from build123d import *

# Parameters (mm, degrees)
F1_DEPTH = 4
F2_DEPTH = 2


with BuildPart() as f1:
    # F0 (on Top) → F1 (new body)
    with BuildSketch(Plane.XY):
        with BuildLine():
            Line((0, 46), (0, 48.5))
            ThreePointArc((0, 48.5), (-43.2585399295, 21.9305431572), (-39.1209598697, -28.6670629621))
            Line((-39.1209598697, -28.6670629621), (-37.1044155465, -27.1893793042))
            ThreePointArc((-37.1044155465, -27.1893793042), (-41.0287182836, 20.8001027883), (0, 46))
        make_face()
        with BuildLine():
            ThreePointArc((-39.1209598697, -28.6670629621), (-0.384054582, -48.498479379), (38.6620589982, -29.2830188679))
            Line((38.6620589982, -29.2830188679), (36.6691693591, -27.7735849057))
            ThreePointArc((36.6691693591, -27.7735849057), (-0.3642579541, -45.9985577616), (-37.1044155465, -27.1893793042))
            Line((-37.1044155465, -27.1893793042), (-39.1209598697, -28.6670629621))
        make_face()
        with BuildLine():
            ThreePointArc((48.5, 0), (34.2946788875, 34.2946788875), (0, 48.5))
            Line((0, 48.5), (0, 46))
            ThreePointArc((0, 46), (32.5269119346, 32.5269119346), (46, 0))
            ThreePointArc((46, 0), (43.6049411794, -14.6495428168), (36.6691693591, -27.7735849057))
            Line((36.6691693591, -27.7735849057), (38.6620589982, -29.2830188679))
            ThreePointArc((38.6620589982, -29.2830188679), (45.9747749392, -15.445713622), (48.5, 0))
        make_face()
    extrude(amount=F1_DEPTH)

    # F0 (on Top) → F2 (join)
    with BuildSketch(Plane.XY):
        with BuildLine():
            Line((0, 48.5), (0, 50))
            ThreePointArc((-3e-10, 50), (-3.0000000001, 49.9099188539), (-5.9891902625, 49.64))
            ThreePointArc((-5.9891902625, 49.64), (-44.596432917, 22.6088073786), (-43.5805555109, -24.5098996604))
            ThreePointArc((-43.5805555109, -24.5098996604), (-42.0314458226, -27.0805753644), (-40.3308865052, -29.5536731))
            Line((-40.3308864636, -29.5536731568), (-39.1209598697, -28.6670629621))
            ThreePointArc((-39.1209598697, -28.6670629621), (-43.2585399295, 21.9305431572), (0, 48.5))
        make_face()
        with BuildLine():
            Line((0, 45), (0, 46))
            ThreePointArc((0, 46), (-41.0287182836, 20.8001027883), (-37.1044155465, -27.1893793042))
            Line((-37.1044155465, -27.1893793042), (-36.2977978173, -26.5983058411))
            ThreePointArc((-36.2977978173, -26.5983058411), (-40.1367896253, 20.3479266407), (0, 45))
        make_face()
        with BuildLine():
            ThreePointArc((35.9547017982, -34.7456388429), (37.9746633311, -32.5257581755), (39.8577928138, -30.1886792029))
            Line((39.8577927817, -30.1886792453), (38.6620589982, -29.2830188679))
            ThreePointArc((38.6620589982, -29.2830188679), (-0.384054582, -48.498479379), (-39.1209598697, -28.6670629621))
            Line((-39.1209598697, -28.6670629621), (-40.3308864636, -29.5536731568))
            ThreePointArc((-40.3308865052, -29.5536731), (-38.4850050472, -31.9202817425), (-36.5004526513, -34.1718737597))
            ThreePointArc((-36.5004526513, -34.1718737597), (-0.3959325588, -49.9984323495), (35.9547017982, -34.7456388429))
        make_face()
        with BuildLine():
            ThreePointArc((-37.1044155465, -27.1893793042), (-0.3642579541, -45.9985577616), (36.6691693591, -27.7735849057))
            Line((36.6691693591, -27.7735849057), (35.8720135035, -27.1698113208))
            ThreePointArc((35.8720135035, -27.1698113208), (-0.3563393029, -44.9985891146), (-36.2977978173, -26.5983058411))
            Line((-36.2977978173, -26.5983058411), (-37.1044155465, -27.1893793042))
        make_face()
        with BuildLine():
            ThreePointArc((-45.1705928336, -33.1001139433), (-41.0669741282, -35.5083498861), (-36.5004526513, -34.1718737597))
            ThreePointArc((-36.5004526513, -34.1718737597), (-38.4850050472, -31.9202817425), (-40.3308865052, -29.5536731))
            ThreePointArc((-40.3308865052, -29.5536731), (-39.8994627937, -30.3940375655), (-39.7507396514, -31.3268935462))
            ThreePointArc((-39.7507396514, -31.3268935462), (-41.8178836997, -34.1781704134), (-45.1705928336, -33.1001139433))
        make_face()
        with BuildLine():
            ThreePointArc((-39.7507396514, -31.3268935462), (-39.8994627937, -30.3940375655), (-40.3308865052, -29.5536731))
            ThreePointArc((-40.3308865052, -29.5536731), (-44.5239600731, -28.907040382), (-45.1705928336, -33.1001139433))
            ThreePointArc((-45.1705928336, -33.1001139433), (-41.8178836997, -34.1781704134), (-39.7507396514, -31.3268935462))
        make_face()
        with BuildLine():
            ThreePointArc((-40.7507396514, -31.3268935462), (-44.6515908972, -31.948797511), (-41.1375041929, -30.1447466199))
            ThreePointArc((-41.1375041929, -30.1447466199), (-40.8498884057, -30.7049895814), (-40.7507396514, -31.3268935462))
        make_face(mode=Mode.SUBTRACT)
        with BuildLine():
            ThreePointArc((-40.3308865052, -29.5536731), (-42.0314458226, -27.0805753644), (-43.5805555109, -24.5098996604))
            ThreePointArc((-43.5805555109, -24.5098996604), (-46.2306698509, -28.4616310409), (-45.1705928336, -33.1001139433))
            ThreePointArc((-45.1705928336, -33.1001139433), (-44.5239600731, -28.907040382), (-40.3308865052, -29.5536731))
        make_face()
        with BuildLine():
            ThreePointArc((44.640728683, -33.8113197413), (40.4379400794, -34.3914679346), (39.8577928138, -30.1886792029))
            ThreePointArc((39.8577928138, -30.1886792029), (37.9746633311, -32.5257581755), (35.9547017982, -34.7456388429))
            ThreePointArc((35.9547017982, -34.7456388429), (40.4994857112, -36.154266407), (44.640728683, -33.8113197413))
        make_face()
        with BuildLine():
            ThreePointArc((44.640728683, -33.8113197413), (45.774130629, -29.1902071747), (43.1869315491, -25.1970026665))
            ThreePointArc((43.1869315491, -25.1970026665), (41.597304838, -27.7428230397), (39.8577928138, -30.1886792029))
            ThreePointArc((39.8577928138, -30.1886792029), (43.2046653401, -29.1561994968), (45.2492603486, -32))
            ThreePointArc((45.2492603486, -32), (45.0930610627, -32.9554043637), (44.640728683, -33.8113197413))
        make_face()
        with BuildLine():
            ThreePointArc((45.2492603486, -32), (43.2046653401, -29.1561994968), (39.8577928138, -30.1886792029))
            ThreePointArc((39.8577928138, -30.1886792029), (40.4379400794, -34.3914679346), (44.640728683, -33.8113197413))
            ThreePointArc((44.640728683, -33.8113197413), (45.0930610627, -32.9554043637), (45.2492603486, -32))
        make_face()
        with BuildLine():
            ThreePointArc((44.2492603486, -32), (41.6123237043, -33.8958670078), (40.6549486373, -30.7924528302))
            ThreePointArc((40.6549486373, -30.7924528302), (42.8861969928, -30.1041329922), (44.2492603486, -32))
        make_face(mode=Mode.SUBTRACT)
        with BuildLine():
            ThreePointArc((43.1869315491, -25.1970026665), (48.2666892248, -13.050927602), (50, 0))
            ThreePointArc((50, 0), (37.4129624136, 33.1703217265), (5.9891902625, 49.64))
            ThreePointArc((5.9891902625, 49.64), (2.9999999999, 49.9099188539), (-3e-10, 50))
            Line((0, 50), (0, 48.5))
            ThreePointArc((0, 48.5), (34.2946788875, 34.2946788875), (48.5, 0))
            ThreePointArc((48.5, 0), (45.9747749392, -15.445713622), (38.6620589982, -29.2830188679))
            Line((38.6620589982, -29.2830188679), (39.8577927817, -30.1886792453))
            ThreePointArc((39.8577928138, -30.1886792029), (41.597304838, -27.7428230397), (43.1869315491, -25.1970026665))
        make_face()
        with BuildLine():
            ThreePointArc((46, 0), (32.5269119346, 32.5269119346), (0, 46))
            Line((0, 46), (0, 45))
            ThreePointArc((0, 45), (31.8198051534, 31.8198051534), (45, 0))
            ThreePointArc((45, 0), (42.6570076755, -14.3310744947), (35.8720135035, -27.1698113208))
            Line((35.8720135035, -27.1698113208), (36.6691693591, -27.7735849057))
            ThreePointArc((36.6691693591, -27.7735849057), (43.6049411794, -14.6495428168), (46, 0))
        make_face()
        with BuildLine():
            ThreePointArc((0, 56), (-3, 53.0000000001), (-3e-10, 50))
            ThreePointArc((-3e-10, 50), (2.1213203435, 50.8786796564), (3, 53))
            ThreePointArc((3, 53), (2.1213203436, 55.1213203436), (0, 56))
        make_face()
        with BuildLine():
            ThreePointArc((2, 53), (1.4142135624, 51.5857864376), (0, 51))
            ThreePointArc((0, 51), (-1.4142135624, 54.4142135624), (2, 53))
        make_face(mode=Mode.SUBTRACT)
        with BuildLine():
            ThreePointArc((-3e-10, 50), (2.9999999999, 49.9099188539), (5.9891902625, 49.64))
            ThreePointArc((5.9891902625, 49.64), (4.3680659336, 54.1133927602), (0, 56))
            ThreePointArc((0, 56), (2.1213203436, 55.1213203436), (3, 53))
            ThreePointArc((3, 53), (2.1213203435, 50.8786796564), (-3e-10, 50))
        make_face()
        with BuildLine():
            ThreePointArc((-5.9891902625, 49.64), (-3.0000000001, 49.9099188539), (-3e-10, 50))
            ThreePointArc((-3e-10, 50), (-3, 53.0000000001), (0, 56))
            ThreePointArc((0, 56), (-4.3680659336, 54.1133927602), (-5.9891902625, 49.64))
        make_face()
    extrude(amount=F2_DEPTH)


solid = f1.part
Read the model definition and answer for the solid it produces. Units are mm, in the model's axes. A direction names the side the tool comes from. Give positions to 0.01 mm unless a question says otherwise; leave off trailing zeros. Write each loop counter-clockwise with the first axis right and the second up, starting at its lowest first coordinate (ties: lowest second). Pieces come first, ordered by that corner, then holes. Notation, with made-up numbers: M -35,41.25 L 24,41.25 A20 ccw 24,48.25 Z; hole C 62,16 d5. An arc over 180 degrees is marked long. One line per item, written item: value. Start each with the question number.
(1) Find section B-B (x = -31). Determine the outline of the cut face in (y, z), plus the area to 3 significant figures.
(2) Find section A-A (y = 18). Determine the outline of the cut face in (x, z), plus the area to 3 significant figures.
(3) Determine the mould class of faces 1 (the cylindrical face through (-44.28, 23.22, 0.99)), 2 (the cylindrical face through (37.944, 24.192, 0.986)), 3 (the flat face through (29, 36, 4)) for opening direction X: pulls with the +X half, pulls with the -X half, needs draft (parallel to the pull), parting line crosses it, or undercut.
(4) Flat-ended cylindrical pins translate along their axes: pin 1 Ø1.5 at (x, z) = (30, 1) entering from -Y; pin 2 Ø5 at (x, y) = (-42.75, -31.33) entering from -Z; pin 3 Ø2.5 at (x, y) = (0, 53) entering from +Z; pin 4 Ø1.5 at (y, z) = (7, 1) entering from -X. Find the tip coordinate at first contact, or state that the pin passes through.
(5) A tool of negligible diameter and unlimited length cuts with its end or side. For faces 4 (the flat face through (34, -30, 2)), 5 (the cylindrical face through (-0.96, -49.99, 0.99)), from which of +Z, -Z, +X, -X, +Y, -Y can it reach the whole face along a straight path? Write none if from no direction.
(6) Find the intervals of material crossed by line 1 (X direction, y = -32.5, z = 0.4); line 2 (Y direction, x = -2, z = 3.35); line 3 (Y direction, x = 39.5, z = 2.9), in increasing order.
Results below:
1. outline: M -39.23,0 L -32.62,0 L -32.62,2 L -33.99,2 L -33.99,4 L -37.3,4 L -37.3,2 L -39.23,2 Z; M 32.62,0 L 39.23,0 L 39.23,2 L 37.3,2 L 37.3,4 L 33.99,4 L 33.99,2 L 32.62,2 Z
1. area: 39.7 mm^2
2. outline: M -46.65,0 L -41.24,0 L -41.24,2 L -42.33,2 L -42.33,4 L -45.04,4 L -45.04,2 L -46.65,2 Z; M 41.24,0 L 46.65,0 L 46.65,2 L 45.04,2 L 45.04,4 L 42.33,4 L 42.33,2 L 41.24,2 Z
2. area: 32.4 mm^2
3. face 1: pulls with the -X half
3. face 2: undercut
3. face 3: needs draft
4. pin 1: stops at y = -40.55
4. pin 2: stops at z = 0
4. pin 3: passes through
4. pin 4: stops at x = -49.61
5. face 4: +Z
5. face 5: +Z, -Z, -Y
6. line 1: x = -45.56 to -44.37, -41.13 to -31.12, 31.12 to 40.31, 44.19 to 45.39
6. line 2: y = -48.46 to -45.96, 45.96 to 48.46
6. line 3: y = -28.14 to -23.57, 23.57 to 28.14
